Input: dimensioned drawing with shaded views. Units: mm. Origin: part minimum x, y, z. A direction names the side the tool comes from. Give positions to 0.01 mm unless a question says otherwise; leave off trailing zeros. Order: outer loops, then holes, each group sorted by start corner. A loop starts at its lowest first (then second) coordinate and runs counter-clockwise, first axis right, second up. Notation, with made-up numbers: (34.25, -3.5) - (63.25, -3.5) arc R11 ccw to (63.25, 8.5) - close; hole circle Ø5 at (-33.5, 57). An arc over 180 degrees is marked (long way). Use a Markdown table: item, result.
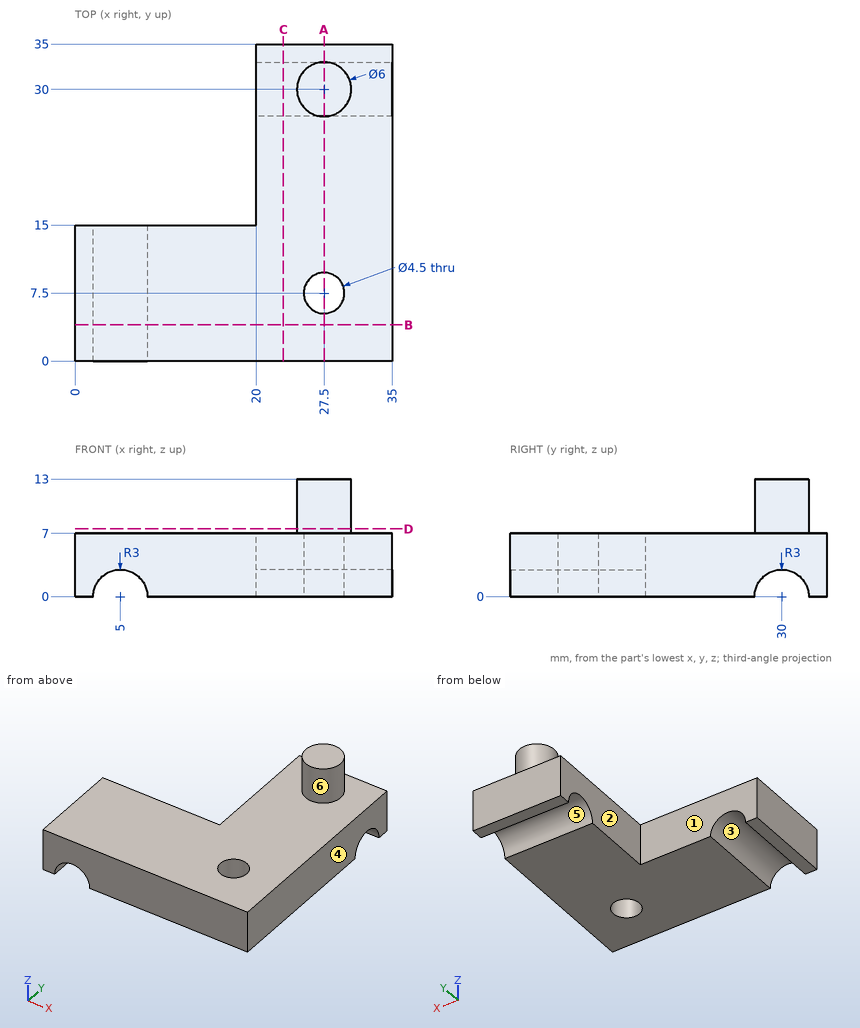
1. Mould query, pull axis X, two halves, no side actions, for the marked faces 1, 2, 3 and 4. Classes: pulls with the +X half, pulls with the -X half, needs draft (parallel to the pull), parting line crosses it, or undercut.
Response:
| item | result |
|---|---|
| face 1 | needs draft |
| face 2 | pulls with the -X half |
| face 3 | undercut |
| face 4 | pulls with the +X half |
2. Pin query (flat end, axial travel): pin 1 (2 mm diameter, centred on x = 30, y = 17, fed in from +Z); pin 2 (2 mm diameter, centred on y = 29.5, z = 4, fed in from -X); pin 3 (2 mm diameter, centred on x = 5, z = 3, fed in from +Y). Return the tip coordinate at first contact, or that it passes through.
Response:
| item | result |
|---|---|
| pin 1 | stops at z = 7 |
| pin 2 | stops at x = 20 |
| pin 3 | stops at y = 15 |
3. Section query D-D (z = 7.5). Return loops of the section in (x, y), then the cut area to 3 significant figures.
Response:
| item | result |
|---|---|
| outline | circle Ø6 at (27.5, 30) |
| area | 28.3 mm^2 |
4. Section query A-A (x = 27.5). Return loops of the section in (y, z), then the cut area to 3 significant figures.
Response:
| item | result |
|---|---|
| outline | (0, 0) - (5.25, 0) - (5.25, 7) - (0, 7) - close; (9.75, 0) - (27, 0) arc R3 cw to (33, 0) - (35, 0) - (35, 7) - (33, 7) - (33, 13) - (27, 13) - (27, 7) - (9.75, 7) - close |
| area | 235 mm^2 |
5. Set-up query: the marked faces 5 and 6. Return all of +Z, -Z, +X, -X, +Y, -Y with unobstructed straight access to the full face (end or side cutting, diameter ignored); none if empty.
Response:
| item | result |
|---|---|
| face 5 | -Z, +X, -X |
| face 6 | +Z |
6. Section query C-C (x = 23). Return loops of the section in (y, z).
Response:
| item | result |
|---|---|
| outline | (0, 0) - (27, 0) arc R3 cw to (33, 0) - (35, 0) - (35, 7) - (0, 7) - close |
7. Material intervals for line 1 along Y through (x, z) = (27.5, 3.5); line 2 along Z through (x, y) = (16.5, 9); line 3 along Y through (x, z) = (15, 5.25), sorted ascending.
Response:
| item | result |
|---|---|
| line 1 | y = 0 to 5.25, 9.75 to 35 |
| line 2 | z = 0 to 7 |
| line 3 | y = 0 to 15 |
8. Section query B-B (y = 4). Return loops of the section in (x, z), then the cut area to 3 significant figures.
Response:
| item | result |
|---|---|
| outline | (0, 0) - (2, 0) arc R3 cw to (8, 0) - (35, 0) - (35, 7) - (0, 7) - close |
| area | 231 mm^2 |
